from build123d import *

# Parameters (mm, degrees)
SKETCH1_W                      = 80
SKETCH1_H                      = 12
SKETCH2_R                      = 60
BOSS_EXTRUDE1_DEPTH            = 11
F_8_4_8_4_DIAMETER_HOLE1_D     = 8.4
F_8_4_8_4_DIAMETER_HOLE1_DEPTH = 23
M100_CLEARANCE_HOLE1_D         = 104


with BuildPart() as part:
    # Sketch1 → Revolve1 (revolve)
    with BuildSketch(Plane.XZ, mode=Mode.PRIVATE) as revolve1_sk:
        with Locations((40, -6)):
            Rectangle(SKETCH1_W, SKETCH1_H)
    revolve(revolve1_sk.sketch.rotate(Axis((0, 0, 0), (0, 0, -1)), 180), axis=Axis((0, 0, 0), (0, 0, -1)))

    # Sketch2 → Boss-Extrude1 (add)
    with BuildSketch(Plane.XY):
        Circle(SKETCH2_R)
    extrude(amount=BOSS_EXTRUDE1_DEPTH)

    # Ø8.4 (8.4) Diameter Hole1
    with Locations(Plane(origin=(0, 0, -12), x_dir=(-1, 0, 0), z_dir=(0, 0, -1))):
        with Locations((21.476681109, 66.098427883), (56.226681109, 40.851075034), (69.5, 0), (56.226681109, -40.851075034), (21.476681109, -66.098427883), (-21.476681109, -66.098427883), (-56.226681109, -40.851075034), (-69.5, 0), (-56.226681109, 40.851075034), (-21.476681109, 66.098427883)):
            Hole(F_8_4_8_4_DIAMETER_HOLE1_D / 2, depth=F_8_4_8_4_DIAMETER_HOLE1_DEPTH)

    # M100 Clearance Hole1 (through all)
    with Locations(Plane(origin=(0, 0, -12), x_dir=(-1, 0, 0), z_dir=(0, 0, -1))):
        with Locations((0, 0)):
            Hole(M100_CLEARANCE_HOLE1_D / 2)


solid = part.part
The listing builds one solid part. Answer for the finished solid, in the listing's coordinates (mm). A direction names the side the tool comes from. Give positions to 0.01 mm unless a question says otherwise; leave off trailing zeros. Write each loop counter-clockwise with the first axis right and the second up, starting at its lowest first coordinate (ties: lowest second). Pieces come first, ordered by that corner, then holes.
1) Find the intervals of material crossed by L1, parallel to Y at x = 0, z = -2.5; L2, parallel to X at y = 67, z = -7.5; L3, parallel to X at y = 17, z = 6.5, in increasing order.
2) Section A-A (y = 0) is taken. Write down the section's boundary in (x, z), and give its area (3 significant figures).
3) Given P1, Ø1, axis at x = 8.5, z = 2.5, coming from the -Y side; P2, Ø5, axis at x = -69.5, y = 0, coming from the -Z side; P3, Ø2, axis at x = -10, z = 3, coming from the -Y side; P4, Ø12, axis at x = -48.5, z = -8, coming from the -Y side, each flat-ended and moving along its own axis, determine where each tip first touches the part or whether it passes through.
4) Section D-D (z = -8.25) is taken. Count the separate pieces of the cut face and the enclosed holes in it, and give its area (3 significant figures).
5) A tool of negligible diameter and unlimited length cuts with its end or side. For faces 1 (the face through (-22.387, -70.199, -5.916)), 2 (the face through (29, -53, 0)), from which of +Z, -Z, +X, -X, +Y, -Y can it reach the whole face along a straight path? Write none if from no direction.
6) Section C-C (y = 57) is taken. Write down the section's boundary in (x, z) (3 decimals).
7) For a pull along Y with two mould halves and no side action, classify faces 3 (the face through (23.415, -69.825, -5.916)), 4 (the face through (52.2, 1.1, -12)), 5 (the face through (-59.94, 2.64, 5.42)) as pulls with the +Y half, pulls with the -Y half, needs draft (parallel to the pull), parting line crosses it, or undercut.
8) Section B-B (x = 0) is taken. Write down the section's boundary in (y, z).
Response:
1. L1: y = -80 to -52, 52 to 80
1. L2: x = -43.71 to -25.58, -17.37 to 17.37, 25.58 to 43.71
1. L3: x = -57.54 to -49.14, 49.14 to 57.54
2. outline: (-80, -12) - (-73.7, -12) - (-73.7, 0) - (-80, 0) - close; (-65.3, -12) - (-52, -12) - (-52, 11) - (-60, 11) - (-60, 0) - (-65.3, 0) - close; (52, -12) - (65.3, -12) - (65.3, 0) - (60, 0) - (60, 11) - (52, 11) - close; (73.7, -12) - (80, -12) - (80, 0) - (73.7, 0) - close
2. area: 646 mm2
3. P1: stops at y = -59.46
3. P2: passes through
3. P3: stops at y = -59.32
3. P4: stops at y = -67.78
4. separate pieces: 1
4. enclosed holes: 11
4. area: 11,100 mm2
5. face 1: +Z, -Z
5. face 2: +Z
6. outline: (-56.134, -12) - (56.134, -12) - (56.134, 0) - (18.735, 0) - (18.735, 11) - (-18.735, 11) - (-18.735, 0) - (-56.134, 0) - close
7. face 3: undercut
7. face 4: needs draft
7. face 5: parting line crosses it
8. outline: (-80, -12) - (-52, -12) - (-52, 11) - (-60, 11) - (-60, 0) - (-80, 0) - close; (52, -12) - (80, -12) - (80, 0) - (60, 0) - (60, 11) - (52, 11) - close
